Geometry check sheet. Reference: the model listing, model coordinates, mm. A direction names the side the tool comes from. Round coordinates to 2 decimals unless told otherwise and drop trailing zeros. Loops run counter-clockwise (first coordinate to the right, second up) from the corner with the lowest first, then second, coordinate; pieces in that order, holes last. Notation, with made-up numbers: M 66,5.25 L 70,5.25 A11 ccw 70,16.25 Z; hole C -4,56 d1. An arc over 180 degrees is marked long. Write item = value, one per line.
from build123d import *

# Parameters (mm, degrees)
F1_DEPTH = 2420
F2_W     = 6
F2_H     = 153
F2_W_2   = 72
F2_H_2   = 178
F3_DEPTH = 165.001
F4_W     = 37.5
F4_H     = 37
F4_H_2   = 3
F4_H_3   = 40
F5_DEPTH = 125.501


with BuildPart() as f1:
    # F0 (on Top) → F1 (new body)
    with BuildSketch(Plane.XY):
        with BuildLine():
            Line((-54, 0), (0, 0))
            Line((0, 0), (0, 4.5))
            Line((0, 4.5), (-49.5, 4.5))
            ThreePointArc((-49.5, 4.5), (-53.7426406871, 6.2573593129), (-55.5, 10.5))
            Line((-55.5, 10.5), (-55.5, 130.6311523413))
            ThreePointArc((-55.5, 130.6311523413), (-54.060089269, 134.5305863848), (-50.4314713804, 136.5584081202))
            Line((-50.4314713804, 136.5584081202), (48.5685286196, 152.1163104777))
            ThreePointArc((48.5685286196, 152.1163104777), (53.3994340434, 150.7491439679), (55.5, 146.1890546989))
            Line((55.5, 146.1890546989), (55.5, 127))
            ThreePointArc((55.5, 127), (57.2573593129, 122.7573593129), (61.5, 121))
            Line((61.5, 121), (105, 121))
            Line((105, 121), (105, 125.5))
            Line((105, 125.5), (66, 125.5))
            ThreePointArc((66, 125.5), (61.7573593129, 127.2573593129), (60, 131.5))
            Line((60, 131.5), (60, 151.4514598279))
            ThreePointArc((60, 151.4514598279), (57.8994340434, 156.0115490969), (53.0685286196, 157.3787156068))
            Line((53.0685286196, 157.3787156068), (-54.9314713804, 140.4064584894))
            ThreePointArc((-54.9314713804, 140.4064584894), (-58.560089269, 138.378636754), (-60, 134.4792027106))
            Line((-60, 134.4792027106), (-60, 6))
            ThreePointArc((-60, 6), (-58.2426406871, 1.7573593129), (-54, 0))
        make_face()
    extrude(amount=F1_DEPTH)

    # F2 (on face) → F3 (cut, through all)
    with BuildSketch(Plane(origin=(-60, 0, 0), x_dir=(0, -1, 0), z_dir=(-1, 0, 0))):
        Polygon((-117.5, 153), (-117.5, 0), (-6, 0), (-6, 153), (-78, 153), align=None)
        with Locations((-3, 76.5)):
            Rectangle(F2_W, F2_H)
        with Locations((-42, 242)):
            Rectangle(F2_W_2, F2_H_2)
        with Locations((-3, 242)):
            Rectangle(F2_W, F2_H_2)
        with Locations((-42, 2178)):
            Rectangle(F2_W_2, F2_H_2)
        with Locations((-3, 2178)):
            Rectangle(F2_W, F2_H_2)
        Polygon((-6, 2420), (-117.5, 2420), (-117.5, 2267), (-78, 2267), (-6, 2267), align=None)
        with Locations((-3, 2343.5)):
            Rectangle(F2_W, F2_H)
    extrude(amount=-F3_DEPTH, mode=Mode.SUBTRACT)

    # F4 (on face) → F5 (cut, through all)
    with BuildSketch(Plane(origin=(0, 125.5, 0), x_dir=(-1, 0, 0), z_dir=(0, 1, 0))):
        with Locations((-86.25, 2398.5)):
            Rectangle(F4_W, F4_H)
        with Locations((-86.25, 2418.5)):
            Rectangle(F4_W, F4_H_2)
        with Locations((-86.25, 20)):
            Rectangle(F4_W, F4_H_3)
    extrude(amount=-F5_DEPTH, mode=Mode.SUBTRACT)


solid = f1.part
(1) Depth check by flat-ended pin: pin 1 Ø1 at (y, z) = (41, 831) entering from +X; pin 2 Ø18 at (x, y) = (-41, 36) entering from -Z; pin 3 Ø5 at (x, y) = (81.5, 123) entering from -Z; pin 4 Ø3.5 at (x, z) = (-58, 201.5) entering from -Y. Enter the tip coordinate at first touch or a pass-through.
Result set:
pin_1 = -55.5
pin_2 = through
pin_3 = 40
pin_4 = 78
(2) Material ranges on line 1 along X through (y, z) = (69.5, 1146); line 2 along X through (y, z) = (132, 2282.5); line 3 along X through (y, z) = (127, 777), recorded low to high. Write a range as from..to.
Result set:
line_1 = -60..-55.5
line_2 = -60..-55.34, 55.5..60
line_3 = -60..-55.5, 55.5..62.03
(3) Sectioned sample at A-A on z = 1947.5. Record the cut outline in (x, y).
Result set:
outline = M -60,6 A6 ccw -54,0 L 0,0 L 0,4.5 L -49.5,4.5 A6 cw -55.5,10.5 L -55.5,130.63 A6 cw -50.43,136.56 L 48.57,152.12 A6 cw 55.5,146.19 L 55.5,127 A6 ccw 61.5,121 L 105,121 L 105,125.5 L 66,125.5 A6 cw 60,131.5 L 60,151.45 A6 ccw 53.07,157.38 L -54.93,140.41 A6 ccw -60,134.48 Z
(4) Sectioned sample at B-B on x = -27. Record the cut outline in (y, z).
Result set:
outline = M 0,331 L 4.5,331 L 4.5,2089 L 0,2089 Z; M 140.24,0 L 144.8,0 L 144.8,2420 L 140.24,2420 Z
(5) Sectioned sample at C-C on y = 41. Record the cut outline in (x, z), then the cut area to 3 significant figures.
Result set:
outline = M -60,331 L -55.5,331 L -55.5,2089 L -60,2089 Z
area = 7,910 mm2
(6) Release check for a two-part mould opening along Y. For faces 5 (the flat face through (83, 121, 1193)), 6 (the flat face through (-57, 21, 331)), 7 (the flat face through (-55.5, 70, 1193)) record: released by +Y, released by -Y, zero draft, split by the parting line, or undercut.
Result set:
face_5 = released by -Y
face_6 = zero draft
face_7 = undercut
(7) Tool access check on faces 1 (the flat face through (-57, 28, 2089)), 2 (the flat face through (-1.62, 144.23, 1193.06)), 3 (the flat face through (-24, 4.5, 1198)), 4 (the flat face through (86, 125.5, 1193)). Record the directions out of +Z, -Z, +X, -X, +Y, -Y that give a thin tool (end or side, any length) a straight path to the whole face; none if there is none.
Result set:
face_1 = +Z, +X, -X, -Y
face_2 = +Z, -Z
face_3 = +Z, -Z, +X
face_4 = +Z, -Z, +X, +Y
